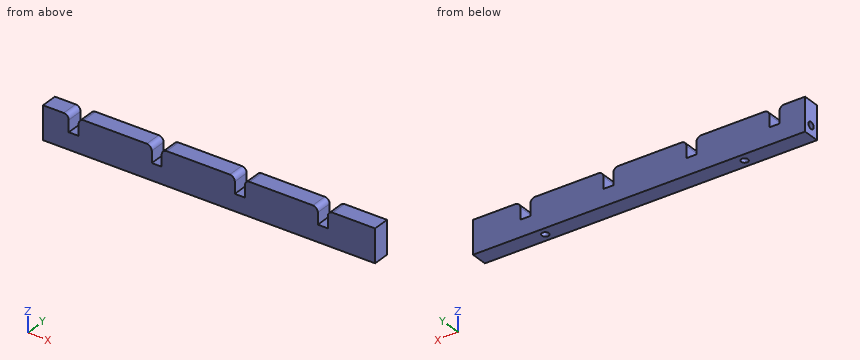
```python
from build123d import *

# Parameters (mm, degrees)
F0_W           = 127
F0_H           = 6.35
F1_DEPTH       = 12.7
F2_W           = 3.81
F2_H           = 6.35
F3_DEPTH       = 6.35
F4_R           = 1.905
F7_D           = 2.7051
F7_DEPTH       = 11.684
F7_TIP         = 0.8126940303
F7_ON_F6_D     = 2.7051
F7_ON_F6_DEPTH = 11.684
F7_ON_F6_TIP   = 0.8126940303


with BuildPart() as f1:
    # F0 (on Top) → F1 (new body)
    with BuildSketch(Plane.XY):
        Rectangle(F0_W, F0_H)
    extrude(amount=F1_DEPTH)

    # F2 (on face) → F3 (cut, through all)
    with BuildSketch(Plane.XZ.offset(3.175)):
        with Locations((-51.7525, 9.525)):
            Rectangle(F2_W, F2_H)
        with Locations((-20.0025, 9.525)):
            Rectangle(F2_W, F2_H)
        with Locations((11.7475, 9.525)):
            Rectangle(F2_W, F2_H)
        with Locations((43.4975, 9.525)):
            Rectangle(F2_W, F2_H)
    extrude(amount=-F3_DEPTH, mode=Mode.SUBTRACT)

    # F4
    f4_edges = [f1.edges().sort_by_distance(p)[0] for p in [
        (-53.6575, 0, 12.7),
        (-49.8475, 0, 12.7),
        (-21.9075, 0, 12.7),
        (-18.0975, 0, 12.7),
        (9.8425, 0, 12.7),
        (13.6525, 0, 12.7),
        (41.5925, 0, 12.7),
        (45.4025, 0, 12.7),
    ]]
    fillet(f4_edges, radius=F4_R)

    # F7
    with Locations(Plane(origin=(0, 0, 0), x_dir=(1, 0, 0), z_dir=(0, 0, -1))):
        with Locations((-38.1, 0), (38.1, 0)):
            Hole(F7_D / 2, depth=F7_DEPTH)
            with Locations((0, 0, -(F7_DEPTH + F7_TIP / 2))):  # 118° drill point
                Cone(0, F7_D / 2, F7_TIP, mode=Mode.SUBTRACT)

    # F7 on F6
    with Locations(Plane(origin=(-63.5, 0, 0), x_dir=(0, -1, 0), z_dir=(-1, 0, 0))):
        with Locations((0, 3.81)):
            Hole(F7_ON_F6_D / 2, depth=F7_ON_F6_DEPTH)
            with Locations((0, 0, -(F7_ON_F6_DEPTH + F7_ON_F6_TIP / 2))):  # 118° drill point
                Cone(0, F7_ON_F6_D / 2, F7_ON_F6_TIP, mode=Mode.SUBTRACT)


solid = f1.part
```
The listing builds one solid part. Answer for the finished solid, in the listing's coordinates (mm). Round coordinates to 2 decimals unless told otherwise and drop trailing zeros. Write each loop counter-clockwise with the first axis right and the second up, starting at its lowest first coordinate (ties: lowest second). Pieces come first, ordered by that corner, then holes. Notation, with made-up numbers: (82, 50) -> (128, 50) arc R22 cw to (128, 65) -> close; hole circle Ø6 at (-5.75, 45.25). An arc over 180 degrees is marked (long way). Write item = value, one per line.
1) Given pin 1 (1.1 mm diameter, centred on x = -51.5, y = 0, fed in from +Z), flat-ended and moving along its own axis, determine where the tip first touches the part or whether it passes through.
Check values:
pin_1 = 6.35
2) Straight lines are drawn through the part: line 1 along X through (y, z) = (2.75, 6.5); line 2 along X through (y, z) = (-2.25, 12); line 3 along Y through (x, z) = (-55.75, 3.81) (3 decimals). For each, find the intervals that lie inside material, in ascending order. Write a range as [from, to].
Check values:
line_1 = [-63.5, -53.66], [-49.85, -21.91], [-18.1, 9.84], [13.65, 41.59], [45.4, 63.5]
line_2 = [-63.5, -54.09], [-49.42, -22.34], [-17.67, 9.41], [14.08, 41.16], [45.83, 63.5]
line_3 = [-3.175, -1.353], [1.353, 3.175]
3) Section A-A on z = 9.5 is taken. Write down the section's boundary in (x, y) (1 decimal).
Check values:
outline = (-63.5, -3.2) -> (-53.7, -3.2) -> (-53.7, 3.2) -> (-63.5, 3.2) -> close; (-49.8, -3.2) -> (-21.9, -3.2) -> (-21.9, 3.2) -> (-49.8, 3.2) -> close; (-18.1, -3.2) -> (9.8, -3.2) -> (9.8, 3.2) -> (-18.1, 3.2) -> close; (13.7, -3.2) -> (41.6, -3.2) -> (41.6, 3.2) -> (13.7, 3.2) -> close; (45.4, -3.2) -> (63.5, -3.2) -> (63.5, 3.2) -> (45.4, 3.2) -> close; hole circle Ø2.7 at (-38.1, 0); hole circle Ø2.7 at (38.1, 0)
